Part model, mm, in its own coordinate system. Face numbers are marked on the shaded views. A direction names the side the tool comes from. Coordinates: 2 decimals unless noted, no trailing zeros. Loops run counter-clockwise (first coordinate to the right, second up) from the corner with the lowest first, then second, coordinate; pieces in that order, holes last. Notation, with made-up numbers: M 47.5,63.5 L 65.5,63.5 A17 ccw 65.5,79.5 Z; hole C -6,-16.5 d4. An arc over 180 degrees is marked long. Use a Markdown table: item, result. Add a question column.
1) Band-saw the part on A-A (y = 0). List the corners of the cut face in (x, z), plus the area to 3 significant figures.
2) Tool access for the marked faces 1 and 2: list every direction of +Z, -Z, +X, -X, +Y, -Y with a clear straight run to the whole face (end or side of a thin tool).
3) Pull direction Y, two halves, no side cores. Call the marked faces 3, 4 and 5: released by +Y, released by -Y, zero draft, split by the parting line, or undercut.
4) Wall check: probe 1 along Y at (x, z) = (-0.75, -7); probe 2 along X at (y, z) = (-0.05, 5); probe 3 along Z at (x, y) = (-4, -0.1). Give the ranges that are in metal, low to high. Write a range as from..to.
5) Band-saw the part on C-C (z = -3). List the corners of the cut face in (x, y).
6) Band-saw the part on B-B (x = -4.5). List the corners of the cut face in (y, z).
7) Pin check, flat tips, straight feed: pin 1 Ø1 at (x, z) = (-7, -1) entering from +Y; pin 2 Ø4 at (x, z) = (-8.5, -2) entering from -Y; pin 3 Ø1.8 at (y, z) = (0, 6.42) entering from +X; pin 4 Ø1.5 at (x, y) = (-4, -0.5) entering from -Z. Stop position of each tip, or through.
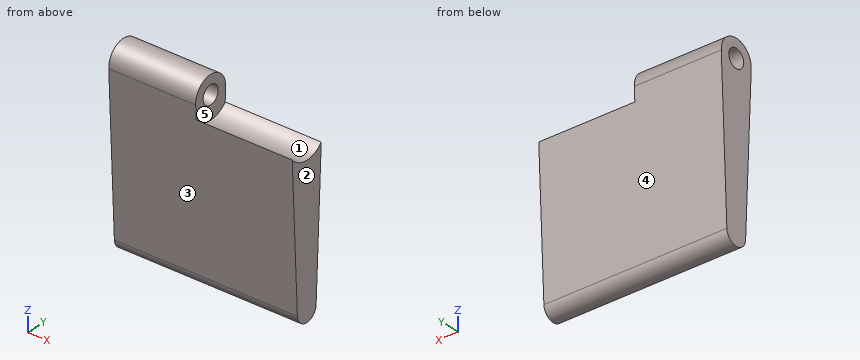
from build123d import *

# Parameters (mm, degrees)
SKETCH1_R           = 0.78486
BOSS_EXTRUDE1_DEPTH = 15.68196
SKETCH2_R           = 1.96088
CUT_EXTRUDE1_DEPTH  = 8.23214


with BuildPart() as part:
    # Sketch1 → Boss-Extrude1 (new body)
    with BuildSketch(Plane(origin=(0, 0, 0), x_dir=(0, 0, -1), z_dir=(1, 0, 0))):
        with BuildLine():
            Line((-6.346883091, -1.565695238), (7.109902444, -0.979511121))
            ThreePointArc((7.109902444, -0.979511121), (8.047674463, 0), (7.109902444, 0.979511121))
            Line((7.109902444, 0.979511121), (-6.346883091, 1.565695238))
            ThreePointArc((-6.346883091, 1.565695238), (-7.982265537, 0), (-6.346883091, -1.565695238))
        make_face()
        with Locations((-6.415085537, 0)):
            Circle(SKETCH1_R, mode=Mode.SUBTRACT)
    extrude(amount=-BOSS_EXTRUDE1_DEPTH)

    # Sketch2 → Cut-Extrude1 (cut)
    with BuildSketch(Plane(origin=(0, 0, 0), x_dir=(0, 0, -1), z_dir=(1, 0, 0))):
        with Locations((-6.415085537, 0)):
            Circle(SKETCH2_R)
    extrude(amount=-CUT_EXTRUDE1_DEPTH, mode=Mode.SUBTRACT)


solid = part.part
Entries:
| question | item | result |
|---|---|---|
| 1 | outline | M -15.68,-8.05 L 0,-8.05 L 0,4.45 L -8.23,4.45 L -8.23,5.63 L -15.68,5.63 Z; M -15.68,7.2 L -8.23,7.2 L -8.23,7.98 L -15.68,7.98 Z |
| 1 | area | 211 mm2 |
| 2 | face 1 | +Z, +X |
| 2 | face 2 | +Z, -Z, +X, +Y, -Y |
| 3 | face 3 | released by -Y |
| 3 | face 4 | released by +Y |
| 3 | face 5 | undercut |
| 4 | probe 1 | -0.98..0.98 |
| 4 | probe 2 | -15.68..-8.23 |
| 4 | probe 3 | -8.04..4.46 |
| 5 | outline | M -15.68,-1.16 L 0,-1.16 L 0,1.16 L -15.68,1.16 Z |
| 6 | outline | M -1.51,5.17 L -0.98,-7.11 A0.98 ccw 0.98,-7.11 L 1.51,5.17 A1.96 cw Z |
| 7 | pin 1 | y = 1.27 |
| 7 | pin 2 | y = -1.29 |
| 7 | pin 3 | x = -8.23 |
| 7 | pin 4 | z = -8.05 |
